Read the model definition and answer for the solid it produces. Units are mm, in the model's axes. Coordinates: 2 decimals unless noted, no trailing zeros. Loops run counter-clockwise (first coordinate to the right, second up) from the corner with the lowest first, then second, coordinate; pieces in that order, holes last. Notation, with made-up numbers: M -4,50 L 36,50 A24 ccw 36,74 Z; hole C 70.25,-23 d6. An arc over 180 degrees is marked long. One line per item, written item: value. Start each with the question number.
1. The part is cut by section D-D (z = 3.65). State how many separate pieces and enclosed holes the cut face has, then the cut area to 3 significant figures.
2. The part is cut by section C-C (y = 27). Write down the section's boundary in (x, z), then the cut area to 4 significant figures.
3. Determine the mould class of faces 1 (the face through (-207.73, 111.5, 2.46)), 2 (the face through (-216, 131, 0)) for opening direction Y: +Y half, -Y half, draft (parallel to the pull), parting line (faces both ways), or undercut.
4. Flat-ended cylindrical pins translate along their axes: pin 1 (1.5 mm diameter, centred on y = 113, z = 3.5, fed in from -X); pin 2 (1 mm diameter, centred on x = -261, z = 3, fed in from +Y); pin 3 (2.5 mm diameter, centred on y = 82.5, z = 2, fed in from +X). Find the tip coordinate at first contact, or state that the pin passes through.
5. Consider probe 1 along Y at (x, z) = (-212.5, 2.4); probe 2 along Y at (x, z) = (-359, 3.85); probe 3 along X at (y, z) = (31, 3.1). Determine where each line is inside the solid, lowest interval first.
6. The part is cut by section B-B (x = -212.5). Write down the section's boundary in (y, z).
7. The part is cut by section A-A (y = 99.5). Write down the section's boundary in (x, z).
```python
from build123d import *

# Parameters (mm, degrees)
SKETCH1_W           = 425
SKETCH1_H           = 210
SKETCH1_R           = 5
BOSS_EXTRUDE1_DEPTH = 5
SKETCH2_W           = 70
SKETCH2_H           = 5
SKETCH2_W_2         = 5
SKETCH2_H_2         = 50
CUT_EXTRUDE1_DEPTH  = 5
SKETCH3_W           = 90
SKETCH3_H           = 5
BOSS_EXTRUDE2_DEPTH = 5
SKETCH4_W           = 5
SKETCH4_H           = 70
BOSS_EXTRUDE3_DEPTH = 5
SKETCH5_W           = 5
SKETCH5_H           = 40
SKETCH5_W_2         = 40
SKETCH5_H_2         = 5
CUT_EXTRUDE2_DEPTH  = 5


with BuildPart() as part:
    # Sketch1 → Boss-Extrude1 (new body)
    with BuildSketch(Plane.XY):
        with Locations((-212.5, 105)):
            Rectangle(SKETCH1_W, SKETCH1_H)
        with Locations((-212.5, 110)):
            Circle(SKETCH1_R, mode=Mode.SUBTRACT)
    extrude(amount=BOSS_EXTRUDE1_DEPTH)

    # Sketch2 → Cut-Extrude1 (cut)
    with BuildSketch(Plane(origin=(0, 0, 0), x_dir=(-1, 0, 0), z_dir=(0, 0, -1))):
        with Locations((90, 2.5)):
            Rectangle(SKETCH2_W, SKETCH2_H)
        with Locations((2.5, 45)):
            Rectangle(SKETCH2_W_2, SKETCH2_H_2)
        with Locations((2.5, 165)):
            Rectangle(SKETCH2_W_2, SKETCH2_H_2)
        with Locations((90, 207.5)):
            Rectangle(SKETCH2_W, SKETCH2_H)
        with Locations((335, 207.5)):
            Rectangle(SKETCH2_W, SKETCH2_H)
        with Locations((422.5, 165)):
            Rectangle(SKETCH2_W_2, SKETCH2_H_2)
        with Locations((422.5, 45)):
            Rectangle(SKETCH2_W_2, SKETCH2_H_2)
        with Locations((335, 2.5)):
            Rectangle(SKETCH2_W, SKETCH2_H)
    extrude(amount=-CUT_EXTRUDE1_DEPTH, mode=Mode.SUBTRACT)

    # Sketch3 → Boss-Extrude2 (add)
    with BuildSketch(Plane.XY.offset(5)):
        with Locations((-335, 212.5)):
            Rectangle(SKETCH3_W, SKETCH3_H)
        with Locations((-90, 212.5)):
            Rectangle(SKETCH3_W, SKETCH3_H)
        with Locations((-335, -2.5)):
            Rectangle(SKETCH3_W, SKETCH3_H)
        with Locations((-90, -2.5)):
            Rectangle(SKETCH3_W, SKETCH3_H)
    extrude(amount=-BOSS_EXTRUDE2_DEPTH)

    # Sketch4 → Boss-Extrude3 (add)
    with BuildSketch(Plane.XY.offset(5)):
        with Locations((-427.5, 165)):
            Rectangle(SKETCH4_W, SKETCH4_H)
        with Locations((-427.5, 45)):
            Rectangle(SKETCH4_W, SKETCH4_H)
        with Locations((2.5, 45)):
            Rectangle(SKETCH4_W, SKETCH4_H)
        with Locations((2.5, 165)):
            Rectangle(SKETCH4_W, SKETCH4_H)
    extrude(amount=-BOSS_EXTRUDE3_DEPTH)

    # Sketch5 → Cut-Extrude2 (cut)
    with BuildSketch(Plane.XY.offset(5)):
        with Locations((-240, 110)):
            Rectangle(SKETCH5_W, SKETCH5_H)
        with Locations((-212.5, 82.5)):
            Rectangle(SKETCH5_W_2, SKETCH5_H_2)
        with Locations((-212.5, 137.5)):
            Rectangle(SKETCH5_W_2, SKETCH5_H_2)
        with Locations((-185, 110)):
            Rectangle(SKETCH5_W, SKETCH5_H)
    extrude(amount=-CUT_EXTRUDE2_DEPTH, mode=Mode.SUBTRACT)


solid = part.part
```
Answer block:
1. separate pieces: 1
1. enclosed holes: 13
1. area: 89,200 mm2
2. outline: M -430,0 L -425,0 L -425,5 L -430,5 Z; M -420,0 L -5,0 L -5,5 L -420,5 Z; M 0,0 L 5,0 L 5,5 L 0,5 Z
2. area: 2,125 mm2
3. face 1: undercut
3. face 2: draft
4. pin 1: stops at x = -425
4. pin 2: stops at y = 210
4. pin 3: stops at x = 0
5. probe 1: y = 0 to 80, 85 to 105, 115 to 135, 140 to 210
5. probe 2: y = -5 to 0, 5 to 205, 210 to 215
5. probe 3: x = -430 to -425, -420 to -5, 0 to 5
6. outline: M 0,0 L 80,0 L 80,5 L 0,5 Z; M 85,0 L 105,0 L 105,5 L 85,5 Z; M 115,0 L 135,0 L 135,5 L 115,5 Z; M 140,0 L 210,0 L 210,5 L 140,5 Z
7. outline: M -425,0 L -242.5,0 L -242.5,5 L -425,5 Z; M -237.5,0 L -187.5,0 L -187.5,5 L -237.5,5 Z; M -182.5,0 L 0,0 L 0,5 L -182.5,5 Z
